Geometry check sheet. Reference: the model listing, model coordinates, mm. A direction names the side the tool comes from. Coordinates: 2 decimals unless noted, no trailing zeros. Write each loop counter-clockwise with the first axis right and the second up, starting at its lowest first coordinate (ties: lowest second). Pieces come first, ordered by that corner, then holes. Notation, with made-up numbers: (16, -20.75) -> (23, -20.75) arc R24 ccw to (23, 2.25) -> close; hole circle Ø8 at (84.25, -10). An arc over 180 degrees is marked (long way). Answer in a Markdown table with one row per item. Add a question column.
Q1. Section check C-C, the plane x = -26. Record the boundary of the cut face in (y, z), and give its area (3 significant figures).
Q2. Thickness scan on line 1 (Y direction, x = -11, z = 3.25); line 2 (Z direction, x = -61, y = -36.5); line 3 (X direction, y = -22.5, z = 48.5). Record the ranges inside material, lowest first.
Q3. Section check B-B, the plane z = 36.35. Record the boundary of the cut face in (x, y), and give its area (3 significant figures).
Q4. Section check D-D, the plane x = -64.1. Record the boundary of the cut face in (y, z), and give its area (3 significant figures).
Q5. Section check A-A, the plane x = -41. Record the boundary of the cut face in (y, z), and give its area (3 significant figures).
Q6. Release check for a two-part mould opening along X. For faces 3 (the face through (-89, -25.8, 12.8)), 4 (the face through (-52.558, -25.169, 3.219)), 5 (the face through (-71, 0, 5)) record: pulls with the +X half, pulls with the -X half, needs draft (parallel to the pull), parting line crosses it, or undercut.
Q7. Gauge pin test, flat ends, axial feed: P1, Ø3, axis at x = -79.5, y = -7.5, coming from the -Z side; P2, Ø4.5, axis at x = -11, y = -40.4, coming from the +Z side; P3, Ø8, axis at y = -38.5, z = 46, coming from the +X side; P4, Ø12, axis at x = -84.5, y = -20.5, coming from the +Z side. Record the tip position at first contact, or that the pin passes through.
Q8. Tool access check on faces 1 (the face through (-98.381, -10.514, 23.957)), 2 (the face through (-95.25, -31, 42)). Record the directions out of +Z, -Z, +X, -X, +Y, -Y that give a thin tool (end or side, any length) a straight path to the whole face; none if there is none.
```python
from build123d import *

# Parameters (mm, degrees)
SKETCH1_W                 = 101.6
SKETCH1_H                 = 50.8
BOSS_EXTRUDE1_DEPTH       = 6.35
SKETCH2_R                 = 1.7145
CUT_EXTRUDE1_DEPTH        = 6.35
SKETCH3_R                 = 1.778
CUT_EXTRUDE2_DEPTH        = 6.35
SKETCH4_R                 = 6.35
CUT_EXTRUDE3_DEPTH        = 6.35
CIRPATTERN1_COUNT         = 4
SKETCH5_W                 = 6.35
SKETCH5_H                 = 50.8
BOSS_EXTRUDE2_DEPTH       = 50.8
SKETCH6_R                 = 6.35
CUT_EXTRUDE4_DEPTH        = 6.35
SKETCH7_R                 = 1.778
CUT_EXTRUDE5_DEPTH        = 6.35
CIRPATTERN2_COUNT         = 4
LPATTERN1_COUNT           = 2
LPATTERN1_PITCH           = 38.1
LPATTERN1_COPY_1_SKETCH_R = 1.778
LPATTERN1_COPY_1_DEPTH    = 6.35
LPATTERN1_COPY_2_SKETCH_R = 1.778
LPATTERN1_COPY_2_DEPTH    = 6.35
LPATTERN1_COPY_3_SKETCH_R = 1.778
LPATTERN1_COPY_3_DEPTH    = 6.35
BOSS_EXTRUDE3_DEPTH       = 50.8
FILLET1_R                 = 6.35


with BuildPart() as part:
    # Sketch1 → Boss-Extrude1 (new body)
    with BuildSketch(Plane.XY):
        with Locations((-50.8, -25.4)):
            Rectangle(SKETCH1_W, SKETCH1_H)
    extrude(amount=BOSS_EXTRUDE1_DEPTH)

    # Sketch2 → Cut-Extrude1 (cut)
    with BuildSketch(Plane.XY.offset(6.35)):
        with Locations((-11, -10.400000028)):
            Circle(SKETCH2_R)
        with Locations((-41, -10.400000028)):
            Circle(SKETCH2_R)
        with Locations((-41, -40.399999972)):
            Circle(SKETCH2_R)
        with Locations((-11, -40.399999972)):
            Circle(SKETCH2_R)
        with Locations((-25.999999972, -40.399999972)):
            Circle(SKETCH2_R)
        with Locations((-25.999999972, -10.400000028)):
            Circle(SKETCH2_R)
    extrude(amount=-CUT_EXTRUDE1_DEPTH, mode=Mode.SUBTRACT)

    # Sketch3 → Cut-Extrude2 (cut)
    with BuildSketch(Plane.XY.offset(6.35)):
        with Locations((-26, -15.621)):
            Circle(SKETCH3_R)
    cut_extrude2 = extrude(amount=-CUT_EXTRUDE2_DEPTH, mode=Mode.SUBTRACT)

    # Sketch4 → Cut-Extrude3 (cut)
    with BuildSketch(Plane.XY.offset(6.35)):
        with Locations((-26, -25.4)):
            Circle(SKETCH4_R)
    cut_extrude3 = extrude(amount=-CUT_EXTRUDE3_DEPTH, mode=Mode.SUBTRACT)

    # CirPattern1: Cut-Extrude2 ×4 about axis
    cirpattern1_axis = Axis((-26, -25.4, 0), (0, 0, 1))
    for i in range(1, CIRPATTERN1_COUNT):
        add(cut_extrude2.rotate(cirpattern1_axis, i * 360 / CIRPATTERN1_COUNT), mode=Mode.SUBTRACT)

    # Sketch5 → Boss-Extrude2 (add)
    with BuildSketch(Plane.XY.offset(6.35)):
        with Locations((-98.425, -25.4)):
            Rectangle(SKETCH5_W, SKETCH5_H)
    extrude(amount=BOSS_EXTRUDE2_DEPTH)

    # Sketch6 → Cut-Extrude4 (cut)
    with BuildSketch(Plane(origin=(-95.25, 0, 0), x_dir=(0, 0, -1), z_dir=(1, 0, 0))):
        with Locations((-36.35, -25.4)):
            Circle(SKETCH6_R)
    extrude(amount=-CUT_EXTRUDE4_DEPTH, mode=Mode.SUBTRACT)

    # Sketch7 → Cut-Extrude5 (cut)
    with BuildSketch(Plane(origin=(-95.25, 0, 0), x_dir=(0, 0, -1), z_dir=(1, 0, 0))):
        with Locations((-49.8247, -11.9253)):
            Circle(SKETCH7_R)
    cut_extrude5 = extrude(amount=-CUT_EXTRUDE5_DEPTH, mode=Mode.SUBTRACT)

    # CirPattern2: Cut-Extrude5 ×4 about axis
    cirpattern2_axis = Axis((0, -25.4, 36.35), (1, 0, 0))
    for i in range(1, CIRPATTERN2_COUNT):
        add(cut_extrude5.rotate(cirpattern2_axis, i * 360 / CIRPATTERN2_COUNT), mode=Mode.SUBTRACT)

    # LPattern1: Cut-Extrude3, Cut-Extrude2 ×2
    with Locations(*[(-i * LPATTERN1_PITCH, 0, 0) for i in range(1, LPATTERN1_COUNT)]):
        add(cut_extrude3, mode=Mode.SUBTRACT)
        add(cut_extrude2, mode=Mode.SUBTRACT)

    # LPattern1 copy 1 sketch → LPattern1 copy 1 (cut)
    with BuildSketch(Plane(origin=(-89.5, 0.6, 6.35), x_dir=(0, 1, 0), z_dir=(0, 0, 1))):
        with Locations((-26, -15.621)):
            Circle(LPATTERN1_COPY_1_SKETCH_R)
    extrude(amount=-LPATTERN1_COPY_1_DEPTH, mode=Mode.SUBTRACT)

    # LPattern1 copy 2 sketch → LPattern1 copy 2 (cut)
    with BuildSketch(Plane(origin=(-90.1, -50.8, 6.35), x_dir=(-1, 0, 0), z_dir=(0, 0, 1))):
        with Locations((-26, -15.621)):
            Circle(LPATTERN1_COPY_2_SKETCH_R)
    extrude(amount=-LPATTERN1_COPY_2_DEPTH, mode=Mode.SUBTRACT)

    # LPattern1 copy 3 sketch → LPattern1 copy 3 (cut)
    with BuildSketch(Plane(origin=(-38.7, -51.4, 6.35), x_dir=(0, -1, 0), z_dir=(0, 0, 1))):
        with Locations((-26, -15.621)):
            Circle(LPATTERN1_COPY_3_SKETCH_R)
    extrude(amount=-LPATTERN1_COPY_3_DEPTH, mode=Mode.SUBTRACT)

    # Sketch8 → Boss-Extrude3 (add)
    with BuildSketch(Plane.XZ.offset(50.8)):
        Polygon((-95.25, 6.35), (-95.25, 19.05), (-82.55, 6.35), align=None)
    extrude(amount=-BOSS_EXTRUDE3_DEPTH)

    # Fillet1
    fillet1_edges = [part.edges().sort_by_distance(p)[0] for p in [
        (-98.425, -50.8, 57.15),
        (-98.425, 0, 57.15),
        (0, -50.8, 3.175),
        (0, 0, 3.175),
    ]]
    fillet(fillet1_edges, radius=FILLET1_R)


solid = part.part
```
Calculated:
| question | item | result |
|---|---|---|
| 1 | outline | (-50.8, 0) -> (-42.11, 0) -> (-42.11, 6.35) -> (-50.8, 6.35) -> close; (-38.69, 0) -> (-36.96, 0) -> (-36.96, 6.35) -> (-38.69, 6.35) -> close; (-33.4, 0) -> (-31.75, 0) -> (-31.75, 6.35) -> (-33.4, 6.35) -> close; (-19.05, 0) -> (-17.4, 0) -> (-17.4, 6.35) -> (-19.05, 6.35) -> close; (-13.84, 0) -> (-12.11, 0) -> (-12.11, 6.35) -> (-13.84, 6.35) -> close; (-8.69, 0) -> (0, 0) -> (0, 6.35) -> (-8.69, 6.35) -> close |
| 1 | area | 153 mm² |
| 2 | line 1 | y = -50.8 to -42.11, -38.69 to -12.11, -8.69 to 0 |
| 2 | line 2 | z = 0 to 6.35 |
| 2 | line 3 | x = -101.6 to -95.25 |
| 3 | outline | (-101.6, -50.8) -> (-95.25, -50.8) -> (-95.25, -31.75) -> (-101.6, -31.75) -> close; (-101.6, -19.05) -> (-95.25, -19.05) -> (-95.25, 0) -> (-101.6, 0) -> close |
| 3 | area | 242 mm² |
| 4 | outline | (-50.8, 0) -> (-36.96, 0) -> (-36.96, 6.35) -> (-50.8, 6.35) -> close; (-33.4, 0) -> (-31.75, 0) -> (-31.75, 6.35) -> (-33.4, 6.35) -> close; (-19.05, 0) -> (-17.4, 0) -> (-17.4, 6.35) -> (-19.05, 6.35) -> close; (-13.84, 0) -> (0, 0) -> (0, 6.35) -> (-13.84, 6.35) -> close |
| 4 | area | 197 mm² |
| 5 | outline | (-50.8, 0) -> (-42.11, 0) -> (-42.11, 6.35) -> (-50.8, 6.35) -> close; (-38.69, 0) -> (-12.11, 0) -> (-12.11, 6.35) -> (-38.69, 6.35) -> close; (-8.69, 0) -> (0, 0) -> (0, 6.35) -> (-8.69, 6.35) -> close |
| 5 | area | 279 mm² |
| 6 | face 3 | pulls with the +X half |
| 6 | face 4 | undercut |
| 6 | face 5 | needs draft |
| 7 | P1 | stops at z = 0 |
| 7 | P2 | stops at z = 6.35 |
| 7 | P3 | stops at x = -95.25 |
| 7 | P4 | stops at z = 14.3 |
| 8 | face 1 | +X, -X |
| 8 | face 2 | +Z, +X, +Y, -Y |
